Can you work these out from the model? Positions are in its coordinate system, mm. Face numbers are marked on the shaded views. A direction names the side the tool comes from. Give positions to 0.01 mm unless a question says otherwise; leave off trailing zeros. Loops run counter-clockwise (first coordinate to the right, second up) from the corner with the lowest first, then second, coordinate; pieces in that order, holes last. Notation, with made-up numbers: M -7,9.5 L 39,9.5 A26 cw 39,48.5 Z; hole C -15.5,-18.75 d7. An arc over 180 degrees is marked long. Use CSV: the item, a comma, the result in double quotes.
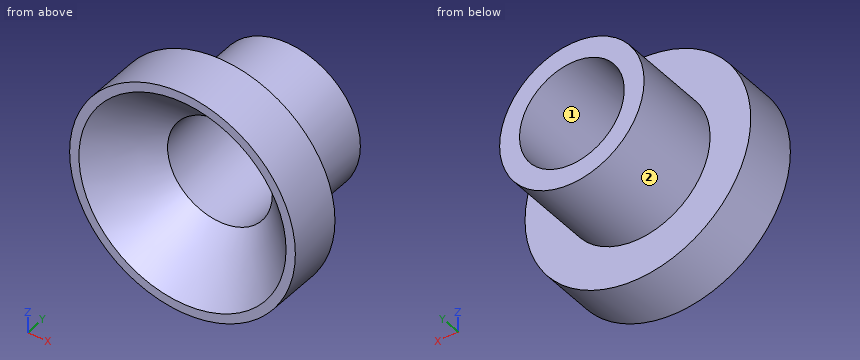
from build123d import *

# Parameters (mm, degrees)
SKETCH1_R                                            = 4
BOSS_EXTRUDE1_DEPTH                                  = 5
SKETCH2_R                                            = 6.25
BOSS_EXTRUDE2_DEPTH                                  = 3
SKETCH3_R                                            = 2.8
CUT_EXTRUDE1_DEPTH                                   = 12.921619018
CSK_FOR_M5_HEX_SOCKET_COUNTERSUNK_HEAD_S_D           = 5.8
CSK_FOR_M5_HEX_SOCKET_COUNTERSUNK_HEAD_S_CSINK_D     = 11.47
CSK_FOR_M5_HEX_SOCKET_COUNTERSUNK_HEAD_S_CSINK_ANGLE = 90


with BuildPart() as part:
    # Sketch1 → Boss-Extrude1 (new body)
    with BuildSketch(Plane(origin=(0, 0, 0), x_dir=(1, 0, 0), z_dir=(0, 1, 0))):
        with Locations(Location((0, 0, 0), (0, 0, 270))):
            Circle(SKETCH1_R)
    extrude(amount=BOSS_EXTRUDE1_DEPTH)

    # Sketch2 → Boss-Extrude2 (add)
    with BuildSketch(Plane.XZ):
        with Locations(Location((0, 0, 0), (0, 0, 270))):
            Circle(SKETCH2_R)
    extrude(amount=BOSS_EXTRUDE2_DEPTH)

    # Sketch3 → Cut-Extrude1 (cut, through all)
    with BuildSketch(Plane(origin=(0, 5, 0), x_dir=(1, 0, 0), z_dir=(0, 1, 0))):
        with Locations(Location((0, 0, 0), (0, 0, 270))):
            Circle(SKETCH3_R)
    extrude(amount=-CUT_EXTRUDE1_DEPTH, mode=Mode.SUBTRACT)

    # CSK for M5 Hex Socket Countersunk Head Screw1 (through all)
    with Locations(Plane(origin=(0, -3, 0), x_dir=(-1, 0, 0), z_dir=(0, -1, 0))):
        with Locations((0, 0)):
            CounterSinkHole(CSK_FOR_M5_HEX_SOCKET_COUNTERSUNK_HEAD_S_D / 2, CSK_FOR_M5_HEX_SOCKET_COUNTERSUNK_HEAD_S_CSINK_D / 2, counter_sink_angle=CSK_FOR_M5_HEX_SOCKET_COUNTERSUNK_HEAD_S_CSINK_ANGLE)


solid = part.part
Q1. For the marked faces 1 and 2, which set-ups out of +Z, -Z, +X, -X, +Y, -Y let a thin tool reach every point of the face, with its end or its side?
Model answer:
face 1,"+Y, -Y"
face 2,"+Y"
Q2. Please list where these lines run through material, in increasing order: L1, parallel to Y at x = 5.25, z = 3; L2, parallel to X at y = 4.5, z = -1.75; L3, parallel to X at y = -2.5, z = 2.25. Write a range as from..to.
Model answer:
L1,"-3..0"
L2,"-3.6..-2.31, 2.31..3.6"
L3,"-5.83..-4.73, 4.73..5.83"
Q3. I want a section at A-A, the plane z = 0. Please give me the cut outline in (x, y) (3 decimals).
Model answer:
outline,"M -6.25,-3 L -5.735,-3 L -2.9,-0.165 L -2.9,5 L -4,5 L -4,0 L -6.25,0 Z; M 2.9,-0.165 L 5.735,-3 L 6.25,-3 L 6.25,0 L 4,0 L 4,5 L 2.9,5 Z"
Q4. I'm going to push flat-ended pins straight in: P1, Ø1.5, axis at x = 4.5, z = 2.5, coming from the -Y side; P2, Ø4.5, axis at x = 0, z = 0, coming from the +Y side; P3, Ø3, axis at y = -1.5, z = 3, coming from the -X side; P4, Ø3, axis at y = 2.5, z = -0.5, coming from the +X side. Where does each tip first touch, or does it pass through?
Model answer:
P1,"y = -3"
P2,"through"
P3,"x = -6.07"
P4,"x = 4"
Q5. I want a section at C-C, the plane y = -1.5. Please give me the cut outline in (x, z) (3 decimals).
Model answer:
outline,"C 0,0 d12.5; hole C 0,0 d8.47"
Q6. I want a section at B-B, the plane x = 0. Please give me the cut outline in (y, z) (3 decimals), then the cut area to 3 significant figures.
Model answer:
outline,"M -3,-6.25 L 0,-6.25 L 0,-4 L 5,-4 L 5,-2.9 L -0.165,-2.9 L -3,-5.735 Z; M -3,5.735 L -0.165,2.9 L 5,2.9 L 5,4 L 0,4 L 0,6.25 L -3,6.25 Z"
area,"23.1 mm2"
